Can you work these out from the model? Positions are in its coordinate system, mm. A direction names the side the tool comes from. Round coordinates to 2 decimals unless told otherwise and drop trailing zeros. Write each loop counter-clockwise with the first axis right and the second up, starting at its lowest first coordinate (ties: lowest second). Pieces come first, ordered by that corner, then holes. Notation, with made-up numbers: (32.25, -37.5) - (62.25, -37.5) arc R27 cw to (62.25, -12.5) - close; hole circle Ø7 at (81, 35.25). An arc over 180 degrees is marked (long way). One line per item, written item: value. Start each with the question number.
(1) I want a section at C-C on y = 47.5. List the corners of the cut face in (x, z) for me, plus the area to 3 significant figures.
(2) On a 3-axis mill with a long thin cutter (end or side, diameter ignored), from which of +Z, -Z, +X, -X, +Y, -Y can I reach the whole of each face in a straight line? I mean faces 5 (the face through (0, 54.5, 8)), 6 (the face through (-55, 15, 2)), 7 (the face through (-1, 57, 5)). Say none if no direction works.
(3) I want a section at A-A on z = 7.25. List the corners of the cut face in (x, y) for me.
(4) I want a section at D-D on x = -34.5. List the corners of the cut face in (y, z) for me.
(5) If I drill on L1, parallel to X at y = 62, z = 0.75; L2, parallel to Y at x = 47, z = 1; L3, parallel to Y at x = -10.5, z = 11.25, over which ranges is the centre line in solid material (lowest first)? Write a range as from..to.
(6) I want a section at B-B on x = 47. List the corners of the cut face in (y, z) for me, plus the area to 3 significant figures.
(7) I'm going to push flat-ended pins straight in: pin 1 Ø1.2 at (x, y) = (8.5, 56.5) entering from +Z; pin 2 Ø3 at (y, z) = (-55.5, 5.5) entering from -X; pin 3 Ø1 at (x, z) = (36, 7) entering from +Y. Where does each tip first touch, or does it pass through?
(8) Thinking about a two-plate mould opening in Y: for faces 1 (the face through (47, -67, 1)), 2 (the face through (-1, 1, 4)), 3 (the face through (55, 15, 2)), 4 (the face through (-47, 60, 1)), which applies, +Y half, -Y half, draft (parallel to the pull), parting line (faces both ways), or undercut?
from build123d import *

# Parameters (mm, degrees)
SKETCH_W     = 114
SKETCH_H     = 114
PAD_DEPTH    = 2
SKETCH001_W  = 109
SKETCH001_H  = 109
PAD001_DEPTH = 2
PAD002_DEPTH = 2
SKETCH003_R  = 2
HOLE_DEPTH   = 4.001
FILLET_R     = 1
SKETCH004_W  = 80
SKETCH004_H  = 2.5
PAD003_DEPTH = 15.5
SKETCH005_W  = 39
SKETCH005_H  = 2.5
PAD004_DEPTH = 10
FILLET001_R  = 1


with BuildPart() as part:
    # Sketch → Pad (new body)
    with BuildSketch(Plane.XY):
        Rectangle(SKETCH_W, SKETCH_H)
    extrude(amount=PAD_DEPTH)

    # Sketch001 (on Face6 of Pad) → Pad001 (join)
    with BuildSketch(Plane.XY.offset(2)):
        Rectangle(SKETCH001_W, SKETCH001_H)
    extrude(amount=PAD001_DEPTH)

    # Sketch002 (on Face5 of Pad001) → Pad002 (join)
    with BuildSketch(Plane.XY.offset(2)):
        with BuildLine():
            ThreePointArc((52, 62), (47, 67), (42, 62))
            Line((42, 62), (42, 57))
            Line((42, 57), (52, 57))
            Line((52, 57), (52, 62))
        make_face()
        with BuildLine():
            ThreePointArc((-42, 62), (-47, 67), (-52, 62))
            Line((-52, 57), (-52, 62))
            Line((-42, 57), (-52, 57))
            Line((-42, 62), (-42, 57))
        make_face()
        with BuildLine():
            ThreePointArc((42, -62), (47, -67), (52, -62))
            Line((52, -57), (52, -62))
            Line((42, -57), (52, -57))
            Line((42, -62), (42, -57))
        make_face()
        with BuildLine():
            ThreePointArc((-52, -62), (-47, -67), (-42, -62))
            Line((-42, -62), (-42, -57))
            Line((-42, -57), (-52, -57))
            Line((-52, -57), (-52, -62))
        make_face()
    extrude(amount=-PAD002_DEPTH)

    # Sketch003 (on Face21 of Pad002) → Hole (cut, through all)
    with BuildSketch(Plane(origin=(0, 0, 0), x_dir=(1, 0, 0), z_dir=(0, 0, -1))):
        with Locations((-47, 62)):
            Circle(SKETCH003_R)
        with Locations((47, 62)):
            Circle(SKETCH003_R)
        with Locations((47, -62)):
            Circle(SKETCH003_R)
        with Locations((-47, -62)):
            Circle(SKETCH003_R)
    extrude(amount=-HOLE_DEPTH, mode=Mode.SUBTRACT)

    # Fillet
    fillet_edges = [part.edges().sort_by_distance(p)[0] for p in [
        (54.5, 54.5, 3),
        (-54.5, 54.5, 3),
        (-54.5, -54.5, 3),
        (54.5, -54.5, 3),
    ]]
    fillet(fillet_edges, radius=FILLET_R)

    # Sketch004 (on Face35 of Fillet) → Pad003 (join)
    with BuildSketch(Plane(origin=(0, 0, 0), x_dir=(1, 0, 0), z_dir=(0, 0, -1))):
        with Locations((0, 55.75)):
            Rectangle(SKETCH004_W, SKETCH004_H)
    extrude(amount=-PAD003_DEPTH)

    # Sketch005 (on Face1 of Pad003) → Pad004 (join)
    with BuildSketch(Plane.XY.offset(2)):
        with Locations((0, 55.75)):
            Rectangle(SKETCH005_W, SKETCH005_H)
    extrude(amount=PAD004_DEPTH)

    # Fillet001
    fillet001_edges = [part.edges().sort_by_distance(p)[0] for p in [
        (57, 57, 1),
        (-57, 57, 1),
        (-57, -57, 1),
        (57, -57, 1),
        (52, 57, 1),
        (52, -57, 1),
        (-42, -57, 1),
        (42, -57, 1),
        (-52, -57, 1),
        (-52, 57, 1),
        (42, 57, 1),
        (-42, 57, 1),
    ]]
    fillet(fillet001_edges, radius=FILLET001_R)


solid = part.part
Established:
1. outline: (-57, 0) - (57, 0) - (57, 2) - (54.5, 2) - (54.5, 4) - (-54.5, 4) - (-54.5, 2) - (-57, 2) - close
1. area: 446 mm2
2. face 5: +Z, +X, -X
2. face 6: +Z, -X
2. face 7: +Z, -Z, +Y
3. outline: (-40, -57) - (40, -57) - (40, -54.5) - (-40, -54.5) - close; (-19.5, 54.5) - (19.5, 54.5) - (19.5, 57) - (-19.5, 57) - close
4. outline: (-57, 0) - (57, 0) - (57, 2) - (54.5, 2) - (54.5, 4) - (-54.5, 4) - (-54.5, 15.5) - (-57, 15.5) - close
5. L1: -52..-49, -45..-42, 42..45, 49..52
5. L2: -67..-64, -60..60, 64..67
5. L3: -57..-54.5, 54.5..57
6. outline: (-67, 0) - (-64, 0) - (-64, 2) - (-67, 2) - close; (-60, 0) - (60, 0) - (60, 2) - (54.5, 2) - (54.5, 4) - (-54.5, 4) - (-54.5, 2) - (-60, 2) - close; (64, 0) - (67, 0) - (67, 2) - (64, 2) - close
6. area: 470 mm2
7. pin 1: z = 12
7. pin 2: x = -40
7. pin 3: y = -54.5
8. face 1: -Y half
8. face 2: undercut
8. face 3: draft
8. face 4: undercut
